Autodesk Inventor part; units mm, degrees
ref_plane "YZ Plane" through (0, 0, 0) normal (1, 0, 0) x (0, 1, 0)
ref_plane "XZ Plane" through (0, 0, 0) normal (0, 1, 0) x (-1, 0, 0)
ref_plane "XY Plane" through (0, 0, 0) normal (0, 0, 1) x (1, 0, 0)
sketch "Sketch1" plane through (0, 0, 0) normal (0, 1, 0) x (-1, 0, 0)
  line L0 (0, 0) -> (-400, 0) construction
  line L1 (-400, 0) -> (-750, 0)
  line L2 (-750, 0) -> (-1050, 0)
  line L3 (-400, 0) -> (-400, -300) construction
  line L4 (-400, -300) -> (-375, -300) construction
  line L5 (-375, -300) -> (-425, -300)
  line L6 (-425, -300) -> (-425, 0)
  line L7 (-425, 0) -> (-375, 0)
  line L8 (-375, 0) -> (-375, -300)
  line L9 (0, 0) -> (-1050, 0)
  line L10 (-1050, 0) -> (-1050, -25)
  line L11 (-1050, -25) -> (0, -25)
  line L12 (0, -25) -> (0, 0)
  arc A0 (0, -25) -> (25, 0) centre (0, 0) ccw
  line L13 (0, 0) -> (25, 0) construction
  line L14 (-750, 0) -> (-750, -150) construction
  line L15 (-750, -150) -> (-725, -150) construction
  line L16 (-725, -150) -> (-775, -150)
  line L17 (-775, -150) -> (-775, 0)
  line L18 (-775, 0) -> (-725, 0)
  line L19 (-725, 0) -> (-725, -150)
  arc A1 (-1075, 0) -> (-1050, -25) centre (-1050, 0) ccw
  line L20 (-1050, 0) -> (-1075, 0)
  line L21 (25, 0) -> (0, 0)
  point P0 (-775, -25)
  point P1 (-725, -25)
  point P2 (-425, -25)
  point P3 (-375, -25)
  dimension "d0" = 400
  dimension "d1" = 350
  dimension "d2" = 300
  dimension "d3" = 300
  dimension "d4" = 25
  dimension "d5" = 50
  dimension "d6" = 1050
  dimension "d7" = 25
  dimension "d8" = 150
  dimension "d9" = 25
  dimension "d10" = 50
revolve "Revolution1" add sketch "Sketch1" angle 360 about axis through (0, 0, 0) along (1, 0, 0)
sketch "Sketch2" plane through (375, 0, 0) normal (-1, 0, 0) x (0, 0, 1)
  circle A0 centre (0, 0) radius 300
  line L0 (0, 300) -> (0, 290)
  line L1 (0, 290) -> (25.5833, 307.4702)
  point P0 (14.1547, 299.6659)
  dimension "d12" = 10
extrude "Extrusion1" cut sketch "Sketch2" against normal blind 284.25 contours A0 L1 L0 picked at (7.8644, 296.5058)
sketch "Sketch3" plane through (775, 0, 0) normal (1, 0, 0) x (0, 0, -1)
  circle A0 centre (0, 0) radius 150
  line L0 (0, 150) -> (0, 140)
  line L1 (0, 140) -> (62.4254, 176.0413)
  point P0 (15.8635, 149.1588)
  dimension "d15" = 10
  dimension "d16" = 60
extrude "Extrusion2" cut sketch "Sketch3" against normal blind 139 contours A0 L1 L0 picked at (8.8167, 146.2616)
sketch "Sketch4" plane through (375, 0, 0) normal (-1, 0, 0) x (0, -0.0235977, 0.9997215)
  line L0 (7.0793, 299.9165) -> (-6.8433, 289.9192)
  line L1 (-6.8433, 289.9192) -> (-7.0793, 299.9165)
  arc A0 (-7.0793, 299.9165) -> (7.0793, 299.9165) centre (0, 0) ccw
  circle A1 centre (0, 0) radius 25
sketch "Sketch5" plane through (425, 0, 0) normal (1, 0, 0) x (0, 0.0235977, -0.9997215)
  line L0 (6.8433, 289.9192) -> (-7.0793, 299.9165)
  arc A0 (-7.0793, 299.9165) -> (7.0793, 299.9165) centre (0, 0) ccw
  line L1 (7.0793, 299.9165) -> (6.8433, 289.9192)
  circle A1 centre (0, 0) radius 25
sketch "Sketch6" plane through (725, 140, 0) normal (-1, 0, 0) x (0, 0, 1)
  line L0 (0, 0) -> (-15.8635, 9.1588)
  arc A0 (-15.8635, 9.1588) -> (0, 10) centre (0, -140) ccw
  line L1 (0, 10) -> (0, 0)
  circle A1 centre (0, -140) radius 25
sketch "Sketch7" plane through (775, 140, 0) normal (1, 0, 0) x (0, 0, -1)
  circle A0 centre (0, -140) radius 25
  line L0 (15.8635, 9.1588) -> (0, 0)
  line L1 (0, 0) -> (0, 10)
  arc A1 (0, 10) -> (15.8635, 9.1588) centre (0, -140) ccw
extrude "Extrusion3" cut sketch "Sketch5" against normal blind 12.5
extrude "Extrusion4" cut sketch "Sketch7" against normal blind 12.5
extrude "Extrusion5" cut sketch "Sketch6" against normal blind 12.5
extrude "Extrusion6" cut sketch "Sketch4" against normal blind 12.5
properties part number "shaft_model_2.5cm" material "Steel"
Build history of the part. All positions in model axes, mm. Round coordinates to 2 decimals unless told otherwise and drop trailing zeros. Write each loop counter-clockwise with the first axis right and the second up, starting at its lowest first coordinate (ties: lowest second). Pieces come first, ordered by that corner, then holes. Notation, with made-up numbers: M 68.25,24.5 L 73.25,24.5 A22 cw 73.25,45.5 Z; hole C 13.25,7.25 d5. An arc over 180 degrees is marked long. Answer in a Markdown table with one row per item.
1. Mould opens along X. For faces 1 (the face through (387.5, -62, -6)), 2 (the face through (737.5, -31, -2)), 3 (the face through (762.5, -31, 2)), 4 (the face through (412.5, -63, 3)) say: +X half, -X half, draft (parallel to the pull), parting line (faces both ways), or undercut.
Geometry check:
| item | result |
|---|---|
| face 1 | -X half |
| face 2 | undercut |
| face 3 | +X half |
| face 4 | undercut |
2. Saw through at B-B (z = -58.5). List the corners of the cut face in (x, y).
Geometry check:
| item | result |
|---|---|
| outline | M 387.5,-294.24 L 412.5,-294.24 L 412.5,294.24 L 387.5,294.24 Z; M 737.5,-138.12 L 762.5,-138.12 L 762.5,138.12 L 737.5,138.12 Z |
3. Probe L1, parallel to X at y = 72, z = -34.5; L2, parallel to X at y = 184, z = -138; L3, parallel to Y at x = 933.5, z = 1. List the from-to ranges inside material, lowest first. Write a range as [from, to].
Geometry check:
| item | result |
|---|---|
| L1 | [387.5, 412.5], [737.5, 762.5] |
| L2 | [387.5, 412.5] |
| L3 | [-24.98, 24.98] |
4. Saw through at C-C (x = 240). List the corners of the cut face in (y, z), and give its area (3 significant figures).
Geometry check:
| item | result |
|---|---|
| outline | C 0,0 d50 |
| area | 1,960 mm2 |
5. Saw through at A-A (y = 108.5). List the corners of the cut face in (x, z).
Geometry check:
| item | result |
|---|---|
| outline | M 387.5,-279.69 L 412.5,-279.69 L 412.5,279.69 L 387.5,279.69 Z; M 737.5,-103.57 L 762.5,-103.57 L 762.5,103.57 L 737.5,103.57 Z |
6. Flat gauge pin, fed straight in: P1, Ø12, axis at y = -217, z = -113.5, coming from the +X side. Where does the tip first touch, or does it go through?
Geometry check:
| item | result |
|---|---|
| P1 | x = 412.5 |
7. Saw through at D-D (z = 236). List the corners of the cut face in (x, y), and give its area (3 significant figures).
Geometry check:
| item | result |
|---|---|
| outline | M 387.5,-185.21 L 412.5,-185.21 L 412.5,185.21 L 387.5,185.21 Z |
| area | 9,260 mm2 |
